Source: CAD feature listing. Evaluate the final solid. Frame: model axes, mm. Face numbers are marked on the shaded views. A direction names the side the tool comes from. Give positions to 0.01 mm unless a question says otherwise; leave off trailing zeros. Order: outer loops, then holes, each group sorted by start corner. A loop starts at its lowest first (then second) coordinate and runs counter-clockwise, first axis right, second up.
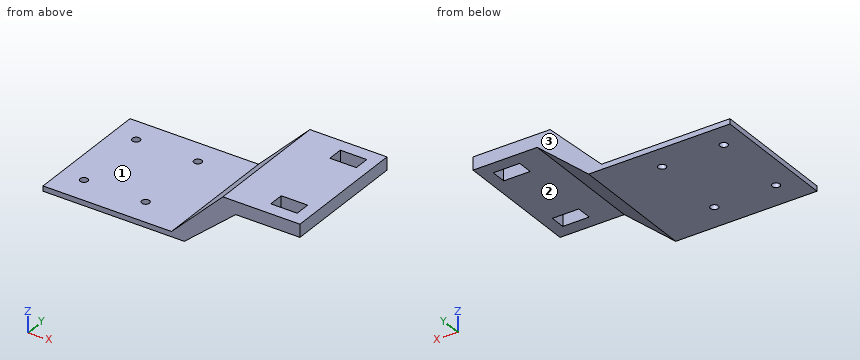
from build123d import *

# Parameters (mm, degrees)
F0_W      = 50
F0_H      = 50
F1_DEPTH  = 2
F2_W      = 25
F2_H      = 50
F3_DEPTH  = 20
F4_W      = 50
F4_H      = 5
F5_DEPTH  = 25
F7_DEPTH  = 50
F8_W      = 3.329061
F8_H      = 5
F8_W_2    = 10.3
F8_H_2    = 6
F9_DEPTH  = 50
F10_W     = 3.329061
F10_H     = 5
F11_DEPTH = 5
F13_DEPTH = 50
F14_W     = 50
F14_H     = 2
F15_DEPTH = 25
F16_R     = 1.5
F17_DEPTH = 50


with BuildPart() as f1:
    # F0 (on Top) → F1 (new body)
    with BuildSketch(Plane.XY):
        with Locations((25, -25)):
            Rectangle(F0_W, F0_H)
    extrude(amount=F1_DEPTH)

    # F2 (on face) → F3 (join)
    with BuildSketch(Plane.XY.offset(2)):
        with Locations((37.5, -25)):
            Rectangle(F2_W, F2_H)
    extrude(amount=F3_DEPTH)

    # F4 (on face) → F5 (join)
    with BuildSketch(Plane.YZ.offset(50)):
        with Locations((-25, 19.5)):
            Rectangle(F4_W, F4_H)
    extrude(amount=F5_DEPTH)

    # F6 (on face) → F7 (cut)
    with BuildSketch(Plane.XZ.offset(50)):
        Polygon((45, 22), (25, 22), (25, 2), align=None)
    extrude(amount=-F7_DEPTH, mode=Mode.SUBTRACT)

    # F8 (on face) → F9 (cut)
    with BuildSketch(Plane(origin=(0, 0, 17), x_dir=(1, 0, 0), z_dir=(0, 0, -1))):
        Polygon((70.513144, 11), (60.213144, 11), (60.213144, 5), (62.5, 5), (65.829061, 5), (70.513144, 5), align=None)
        with Locations((64.16453, 2.5)):
            Rectangle(F8_W, F8_H)
        with Locations((65.336539, 41.898386)):
            Rectangle(F8_W_2, F8_H_2)
    extrude(amount=-F9_DEPTH, mode=Mode.SUBTRACT)

    # F10 (on face) → F11 (join)
    with BuildSketch(Plane(origin=(0, 0, 17), x_dir=(1, 0, 0), z_dir=(0, 0, -1))):
        with Locations((64.16453, 2.5)):
            Rectangle(F10_W, F10_H)
    extrude(amount=-F11_DEPTH)

    # F12 (on face) → F13 (cut)
    with BuildSketch(Plane(origin=(0, 0, 0), x_dir=(-1, 0, 0), z_dir=(0, 1, 0))):
        Polygon((-30, 0), (-50, 17), (-50, 0), align=None)
    extrude(amount=-F13_DEPTH, mode=Mode.SUBTRACT)

    # F14 (on face) → F15 (join)
    with BuildSketch(Plane(origin=(0, 0, 0), x_dir=(0, -1, 0), z_dir=(-1, 0, 0))):
        with Locations((25, 1)):
            Rectangle(F14_W, F14_H)
    extrude(amount=F15_DEPTH)

    # F16 (on face) → F17 (cut)
    with BuildSketch(Plane.XY.offset(2)):
        with Locations((-16.127206, -9.57024)):
            Circle(F16_R)
        with Locations((7.872794, -9.57024)):
            Circle(F16_R)
        with Locations((7.872794, -39.57024)):
            Circle(F16_R)
        with Locations((-16.127206, -39.57024)):
            Circle(F16_R)
    extrude(amount=-F17_DEPTH, mode=Mode.SUBTRACT)


solid = f1.part
1) Section query B-B on x = 42. Output: boundary loops of the cut face in (y, z), and give its area (3 significant figures).
Checks:
outline: (-50, 10.2) - (0, 10.2) - (0, 19) - (-50, 19) - close
area: 440 mm2
2) Section query A-A on y = -31.5. Output: boundary loops of the cut face in (x, z).
Checks:
outline: (-25, 0) - (30, 0) - (50, 17) - (75, 17) - (75, 22) - (45, 22) - (25, 2) - (-25, 2) - close
3) Ray query, L1, parallel to Z at x = -15, y = -33; L2, parallel to X at y = -10, z = 20; L3, parallel to Z at x = 63.5, y = -11.5. Return the intervals inside material, ascending.
Checks:
L1: z = 0 to 2
L2: x = 43 to 60.21, 70.51 to 75
L3: z = 17 to 22
4) Reachability of the marked faces 1, 2 and 3 from +Z, -Z, +X, -X, +Y, -Y: full face, straight path, thin tool, end or side. Return the list, or none.
Checks:
face 1: +Z, -X, +Y, -Y
face 2: -Z, +X, +Y, -Y
face 3: +Z, -Z, +X, -X, +Y
5) Section query C-C on z = 14.5. Output: boundary loops of the cut face in (x, y), and give its area (3 significant figures).
Checks:
outline: (37.5, -50) - (47.06, -50) - (47.06, 0) - (37.5, 0) - close
area: 478 mm2
6) First-contact query: pin 1 Ø1.5 at (x, y) = (21.5, -19) entering from +Z; pin 2 Ø8 at (y, z) = (-31, 8.5) entering from -X; pin 3 Ø4 at (x, y) = (61.5, -13) entering from -Z. Flat tips, straight axial feed; report the tip coordinate or a pass-through.
Checks:
pin 1: stops at z = 2
pin 2: stops at x = 27.5
pin 3: stops at z = 17
